```python
from build123d import *

# Parameters (mm, degrees)
SKETCH006_W     = 114
SKETCH006_H     = 5
PAD002_DEPTH    = 10
SKETCH007_R     = 1.43
POCKET004_DEPTH = 10
CHAMFER001_SIZE = 0.8
SKETCH010_R     = 1.43
POCKET007_DEPTH = 5


with BuildPart() as part:
    # Sketch006 → Pad002 (new body)
    with BuildSketch(Plane.XY):
        with Locations((60, 45)):
            Rectangle(SKETCH006_W, SKETCH006_H)
    extrude(amount=PAD002_DEPTH)

    # Sketch007 (on Face6 of Pad002) → Pocket004 (cut)
    with BuildSketch(Plane.XY.offset(10)):
        with Locations((8, 45)):
            Circle(SKETCH007_R)
        with Locations((112, 45)):
            Circle(SKETCH007_R)
    extrude(amount=-POCKET004_DEPTH, mode=Mode.SUBTRACT)

    # Chamfer001
    chamfer001_edges = [part.edges().sort_by_distance(p)[0] for p in [
        (110.57, 45, 10),
        (6.57, 45, 10),
    ]]
    chamfer(chamfer001_edges, length=CHAMFER001_SIZE)

    # Sketch010 (on Face6 of Chamfer001) → Pocket007 (cut)
    with BuildSketch(Plane.XZ.offset(-42.5)):
        with Locations((75, 5)):
            Circle(SKETCH010_R)
    extrude(amount=-POCKET007_DEPTH, mode=Mode.SUBTRACT)


with BuildPart() as part_1:
    # Body002 placement: moved
    add(part.part.moved(Location((0, 10, 8))))


solid = part_1.part
```
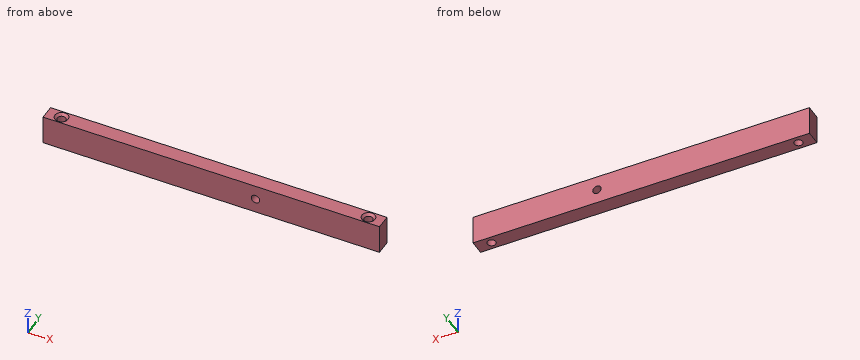
Part model, mm, in its own coordinate system. Coordinates: 2 decimals unless noted, no trailing zeros. Loops run counter-clockwise (first coordinate to the right, second up) from the corner with the lowest first, then second, coordinate; pieces in that order, holes last. Notation, with made-up numbers: (3.5, 8.25) - (24.5, 8.25) arc R11 cw to (24.5, 16.25) - close; hole circle Ø4 at (52, 78.25). An arc over 180 degrees is marked (long way). Write item = value, one per line. Start each with the question number.
Item 1: Flat gauge pin, fed straight in: pin 1 Ø2.5 at (x, y) = (112, 55) entering from -Z. Where does the tip first touch, or does it go through?
Item 2: Cut at B-B, the plane x = 8. Give the cut face in (y, z).
Item 3: Cut at A-A, the plane y = 55. Give the cut face in (x, z), and give its area (3 significant figures).
Item 4: Wall check: L1, parallel to X at y = 55.05, z = 14.5; L2, parallel to Y at x = 8, z = 12.5; L3, parallel to Z at x = 75, y = 53.8. Give the ranges that are in metal, low to high. Write a range as from..to.
Item 5: Cut at C-C, the plane x = 75. Give the cut face in (y, z), and give its area (3 significant figures).
The answers:
q1.pin_1 = through
q2.outline = (52.5, 8) - (53.57, 8) - (53.57, 17.2) - (52.77, 18) - (52.5, 18) - close; (56.43, 8) - (57.5, 8) - (57.5, 18) - (57.23, 18) - (56.43, 17.2) - close
q3.outline = (3, 8) - (6.57, 8) - (6.57, 17.2) - (5.77, 18) - (3, 18) - close; (9.43, 8) - (110.57, 8) - (110.57, 17.2) - (109.77, 18) - (10.23, 18) - (9.43, 17.2) - close; (113.43, 8) - (117, 8) - (117, 18) - (114.23, 18) - (113.43, 17.2) - close; hole circle Ø2.86 at (75, 13)
q3.area = 1,080 mm2
q4.L1 = 3..6.57, 9.43..110.57, 113.43..117
q4.L2 = 52.5..53.57, 56.43..57.5
q4.L3 = 8..11.57, 14.43..18
q5.outline = (52.5, 8) - (57.5, 8) - (57.5, 11.57) - (52.5, 11.57) - close; (52.5, 14.43) - (57.5, 14.43) - (57.5, 18) - (52.5, 18) - close
q5.area = 35.7 mm2
